Job drawing, mm, ordinate dimensions from the low corner. One solid piece. A direction names the side the tool comes from. Round coordinates to 2 decimals unless told otherwise and drop trailing zeros. Loops run counter-clockwise (first coordinate to the right, second up) from the corner with the lowest first, then second, coordinate; pieces in that order, holes last.
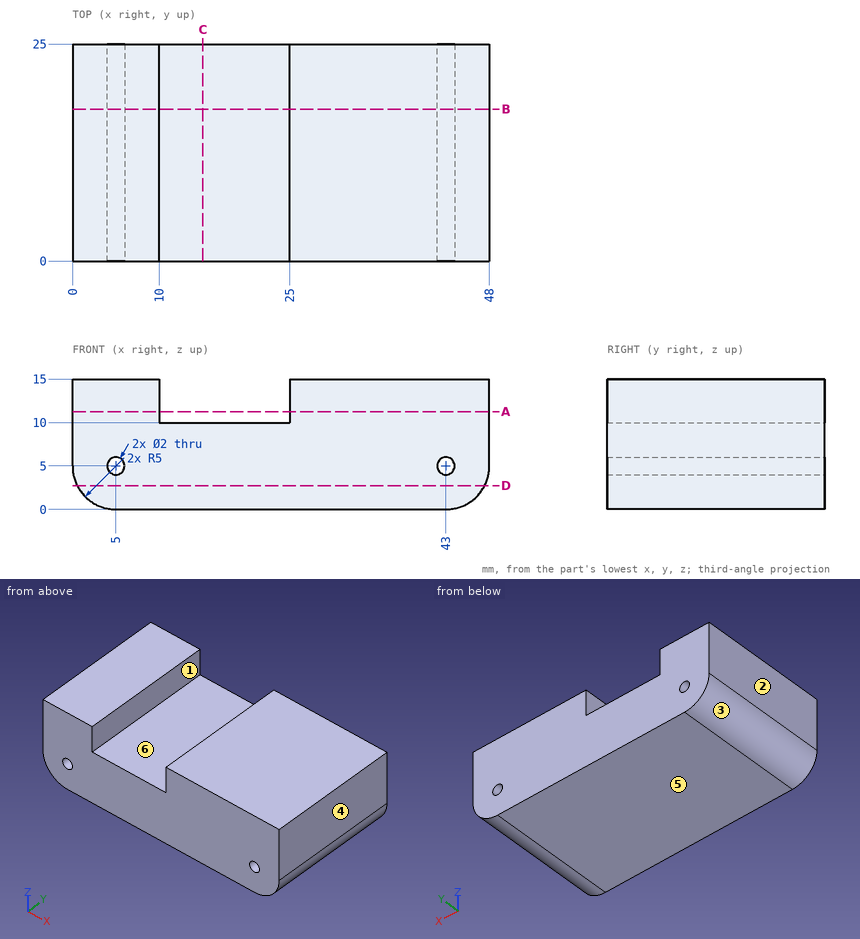
Item 1: Cut at C-C, the plane x = 15. Give the cut face in (y, z).
Answers follow:
outline: (0, 0) - (25, 0) - (25, 10) - (0, 10) - close
Item 2: Two-plate mould, pull along X, no slides. Class the marked faces 3, 4, 5 and 6: released by +X, released by -X, zero draft, split by the parting line, or undercut.
Answers follow:
face 3: released by -X
face 4: released by +X
face 5: zero draft
face 6: undercut
Item 3: Probe line 1 (Z direction, x = 43, y = 8); line 2 (X direction, y = 1.5, z = 5.25); line 3 (X direction, y = 13.75, z = 4.5). List the from-to ranges inside material, lowest first.
Answers follow:
line 1: z = 0 to 4, 6 to 15
line 2: x = 0 to 4.03, 5.97 to 42.03, 43.97 to 48
line 3: x = 0.03 to 4.13, 5.87 to 42.13, 43.87 to 47.97
Item 4: 3-axis set-ups, long thin cutter, end or side, ignore diameter. For the marked faces 1 and 2: which of +Z, -Z, +X, -X, +Y, -Y reach the whole face in a straight line?
Answers follow:
face 1: +Z, +Y, -Y
face 2: +Z, -Z, -X, +Y, -Y
Item 5: Flat gauge pins, fed straight in: P1, Ø1, axis at x = 15, y = 7.5, coming from the +Z side; P2, Ø6, axis at x = 23.5, z = 11, coming from the -Y side; P3, Ø1, axis at y = 15, z = 2.5, coming from the +X side. Where does each tip first touch, or does it go through?
Answers follow:
P1: stops at z = 10
P2: stops at y = 0
P3: stops at x = 47.58
Item 6: Cut at D-D, the plane z = 2.75. Give the cut face in (x, y).
Answers follow:
outline: (0.53, 0) - (47.47, 0) - (47.47, 25) - (0.53, 25) - close
Item 7: Cut at B-B, the plane y = 17.5. Give the cut face in (x, z), plus the area to 3 significant figures.
Answers follow:
outline: (0, 5) arc R5 ccw to (5, 0) - (43, 0) arc R5 ccw to (48, 5) - (48, 15) - (25, 15) - (25, 10) - (10, 10) - (10, 15) - (0, 15) - close; hole circle Ø2 at (5, 5); hole circle Ø2 at (43, 5)
area: 628 mm2
Item 8: Cut at A-A, the plane z = 11.25. Give the cut face in (x, y), plus the area to 3 significant figures.
Answers follow:
outline: (0, 0) - (10, 0) - (10, 25) - (0, 25) - close; (25, 0) - (48, 0) - (48, 25) - (25, 25) - close
area: 825 mm2
